from build123d import *

# Parameters (mm, degrees)
SKETCH1_W           = 37
SKETCH1_H           = 54
BOSS_EXTRUDE1_DEPTH = 2
SKETCH2_W           = 2
SKETCH2_H           = 7
BOSS_EXTRUDE2_DEPTH = 20
CUT_EXTRUDE1_REACH  = 48.626
SKETCH3_R           = 1
SKETCH11_W          = 37
SKETCH11_H          = 54
SKETCH11_W_2        = 33
SKETCH11_H_2        = 50
BOSS_EXTRUDE5_DEPTH = 40
SKETCH12_W          = 134
SKETCH12_H          = 74
BOSS_EXTRUDE6_DEPTH = 2
SKETCH13_W          = 10
SKETCH13_H          = 20
BOSS_EXTRUDE7_DEPTH = 62
CUT_EXTRUDE2_REACH  = 150.084
SKETCH16_R          = 2


with BuildPart() as part:
    # Sketch1 → Boss-Extrude1 (new body)
    with BuildSketch(Plane.XY):
        Rectangle(SKETCH1_W, SKETCH1_H)
    extrude(amount=BOSS_EXTRUDE1_DEPTH)

    # Sketch2 → Boss-Extrude2 (add)
    with BuildSketch(Plane.XY.offset(2)):
        with Locations((13.5, -23.5)):
            Rectangle(SKETCH2_W, SKETCH2_H)
        with Locations((13.5, 23.5)):
            Rectangle(SKETCH2_W, SKETCH2_H)
    extrude(amount=BOSS_EXTRUDE2_DEPTH)

    # Sketch3 → Cut-Extrude1 (cut, up to next)
    with BuildSketch(Plane.ZY.offset(-12.5), mode=Mode.PRIVATE) as cut_extrude1_sk1:
        with Locations((6, -25)):
            Circle(SKETCH3_R)
    cut_extrude1_tool1 = extrude(cut_extrude1_sk1.sketch, amount=-CUT_EXTRUDE1_REACH, mode=Mode.PRIVATE) & part.part
    # Sketch3 → Cut-Extrude1 (cut, up to next)
    with BuildSketch(Plane.ZY.offset(-12.5), mode=Mode.PRIVATE) as cut_extrude1_sk2:
        with Locations((18, -25)):
            Circle(SKETCH3_R)
    cut_extrude1_tool2 = extrude(cut_extrude1_sk2.sketch, amount=-CUT_EXTRUDE1_REACH, mode=Mode.PRIVATE) & part.part
    # Sketch3 → Cut-Extrude1 (cut, up to next)
    with BuildSketch(Plane.ZY.offset(-12.5), mode=Mode.PRIVATE) as cut_extrude1_sk3:
        with Locations((6, 25)):
            Circle(SKETCH3_R)
    cut_extrude1_tool3 = extrude(cut_extrude1_sk3.sketch, amount=-CUT_EXTRUDE1_REACH, mode=Mode.PRIVATE) & part.part
    # Sketch3 → Cut-Extrude1 (cut, up to next)
    with BuildSketch(Plane.ZY.offset(-12.5), mode=Mode.PRIVATE) as cut_extrude1_sk4:
        with Locations((18, 25)):
            Circle(SKETCH3_R)
    cut_extrude1_tool4 = extrude(cut_extrude1_sk4.sketch, amount=-CUT_EXTRUDE1_REACH, mode=Mode.PRIVATE) & part.part
    add(cut_extrude1_tool1.solids().sort_by_distance((12.5, -25, 6))[0], mode=Mode.SUBTRACT)
    add(cut_extrude1_tool2.solids().sort_by_distance((12.5, -25, 18))[0], mode=Mode.SUBTRACT)
    add(cut_extrude1_tool3.solids().sort_by_distance((12.5, 25, 6))[0], mode=Mode.SUBTRACT)
    add(cut_extrude1_tool4.solids().sort_by_distance((12.5, 25, 18))[0], mode=Mode.SUBTRACT)

    # Sketch11 → Boss-Extrude5 (add)
    with BuildSketch(Plane(origin=(0, 0, 0), x_dir=(-1, 0, 0), z_dir=(0, 0, -1))):
        Rectangle(SKETCH11_W, SKETCH11_H)
        Rectangle(SKETCH11_W_2, SKETCH11_H_2, mode=Mode.SUBTRACT)
    extrude(amount=BOSS_EXTRUDE5_DEPTH)

    # Sketch12 → Boss-Extrude6 (add)
    with BuildSketch(Plane(origin=(0, 0, -40), x_dir=(-1, 0, 0), z_dir=(0, 0, -1))):
        with Locations((-48.5, 10)):
            Rectangle(SKETCH12_W, SKETCH12_H)
    extrude(amount=BOSS_EXTRUDE6_DEPTH)

    # Sketch13 → Boss-Extrude7 (add)
    with BuildSketch(Plane.XY.offset(-40)):
        with Locations((110.5, 10)):
            Rectangle(SKETCH13_W, SKETCH13_H)
    extrude(amount=BOSS_EXTRUDE7_DEPTH)

    # Sketch16 → Cut-Extrude2 (cut, up to next)
    with BuildSketch(Plane(origin=(115.5, 0, 0), x_dir=(0, 0, -1), z_dir=(1, 0, 0)), mode=Mode.PRIVATE) as cut_extrude2_sk1:
        with Locations((-12, 10)):
            Circle(SKETCH16_R)
    cut_extrude2_tool1 = extrude(cut_extrude2_sk1.sketch, amount=-CUT_EXTRUDE2_REACH, mode=Mode.PRIVATE) & part.part
    add(cut_extrude2_tool1.solids().sort_by_distance((115.5, 10, 12))[0], mode=Mode.SUBTRACT)


solid = part.part
For this review, take the finished solid that the model builds, in its own axes (mm). A direction names the side the tool comes from. Give positions to 0.01 mm unless a question says otherwise; leave off trailing zeros. Order: outer loops, then holes, each group sorted by start corner. A loop starts at its lowest first (then second) coordinate and runs counter-clockwise, first axis right, second up. Notation, with made-up numbers: (45, 70) - (65, 70) arc R29 cw to (65, 90) - close; hole circle Ø7 at (-30.75, -21.75). An arc over 180 degrees is marked (long way). Answer as a JSON object with one key per item and string values. Group by question number.
Item 1: Take a section at C-C on z = 12. Give the boundary of the cut face in (x, y).
Item 2: Take a section at A-A on z = -9. Give the boundary of the cut face in (x, y).
Item 3: Machinability: for faces 5 (the flat face through (18.5, 0, -19)), 6 (the flat face through (0, 25, -20)), 7 (the flat face through (12.5, -24, 12)), which of the approach directions +Z, -Z, +X, -X, +Y, -Y give a long, thin tool a straight path to every point of the face, cutting with its end or side? Answer none if there is none.
Item 4: Clearance check with flat-ended pins moving along their axes: pin 1 Ø7.5 at (y, z) = (-24, 12.5) entering from +X; pin 2 Ø2 at (y, z) = (27.5, -28.5) entering from -X; pin 3 Ø1.8 at (y, z) = (-25, 18) entering from -X; pin 4 Ø0.6 at (x, z) = (13.5, 8) entering from +Y. State where each tip first meets the part, or that it passes through.
Item 5: Take a section at D-D on y = -18. Give the boundary of the cut face in (x, z).
Item 6: Draft analysis for pull direction Y (two halves, no side actions). For faces 1 (the flat face through (9, -27, -22)), 2 (the flat face through (105.5, 10, -9)), 3 (the flat face through (0, 0, -40)), 4 (the flat face through (0, -25, -20)), state which applies: pulls with the +Y half, pulls with the -Y half, needs draft (parallel to the pull), parting line crosses it, or undercut.
Item 7: Wall thickness on line 1 along Y through (x, z) = (13, 18); line 2 along X through (y, z) = (1, -22.5); line 3 along X through (y, z) = (-9, -12): over which ranges is each line inside the solid? List them lowest first.
Item 8: Take a section at B-B on y = 10. Give the boundary of the cut face in (x, z), and give its area (3 significant figures).
Reported:
{
 "1": {"outline": "(12.5, -27) - (14.5, -27) - (14.5, -20) - (12.5, -20) - close; (12.5, 20) - (14.5, 20) - (14.5, 27) - (12.5, 27) - close; (105.5, 0) - (115.5, 0) - (115.5, 8) - (105.5, 8) - close; (105.5, 12) - (115.5, 12) - (115.5, 20) - (105.5, 20) - close"},
 "2": {"outline": "(-18.5, -27) - (18.5, -27) - (18.5, 27) - (-18.5, 27) - close; (105.5, 0) - (115.5, 0) - (115.5, 20) - (105.5, 20) - close; hole (-16.5, -25) - (16.5, -25) - (16.5, 25) - (-16.5, 25) - close"},
 "3": {"face 5": "+Z, +Y, -Y", "face 6": "none", "face 7": "+Z, -X, +Y, -Y"},
 "4": {"pin 1": "x = 14.5", "pin 2": "x = -18.5", "pin 3": "through", "pin 4": "y = 27"},
 "5": {"outline": "(-18.5, -42) - (115.5, -42) - (115.5, -40) - (18.5, -40) - (18.5, 2) - (-18.5, 2) - close; hole (-16.5, -40) - (16.5, -40) - (16.5, 0) - (-16.5, 0) - close"},
 "6": {"face 1": "pulls with the -Y half", "face 2": "needs draft", "face 3": "undercut", "face 4": "undercut"},
 "7": {"line 1": "-27 to -26, -24 to -20, 20 to 24, 26 to 27", "line 2": "-18.5 to -16.5, 16.5 to 18.5, 105.5 to 115.5", "line 3": "-18.5 to -16.5, 16.5 to 18.5"},
 "8": {"outline": "(-18.5, -42) - (115.5, -42) - (115.5, 10) - (105.5, 10) - (105.5, -40) - (18.5, -40) - (18.5, 2) - (-18.5, 2) - close; (105.5, 14) - (115.5, 14) - (115.5, 22) - (105.5, 22) - close; hole (-16.5, -40) - (16.5, -40) - (16.5, 0) - (-16.5, 0) - close", "area": "1,080 mm^2"}
}
